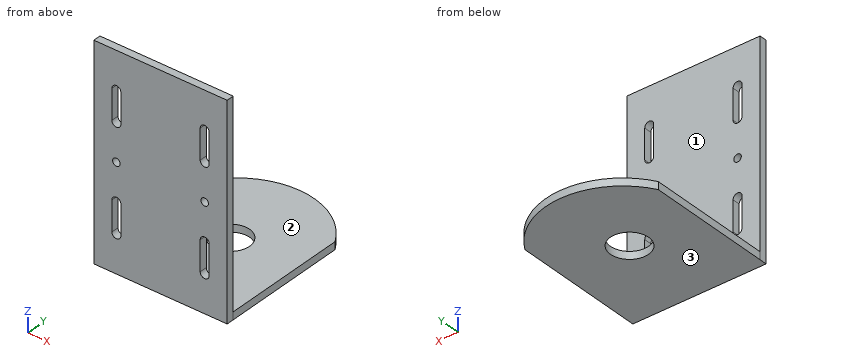
```python
from build123d import *

# Parameters (mm, degrees)
BOSS_EXTRUDE2_DEPTH = 10
BOSS_EXTRUDE3_DEPTH = 10
SKETCH2_R           = 25.4
CUT_EXTRUDE2_DEPTH  = 373.037550256
CUT_EXTRUDE5_DEPTH  = 10
SKETCH4_R           = 5
CUT_EXTRUDE6_DEPTH  = 366.966927049


with BuildPart() as part:
    # 3DSketch1 → Boss-Extrude2 (new body)
    with BuildSketch(Plane(origin=(88.9, 0, 0), x_dir=(-0.5368754921931593, 0, 0.8436614877321076), z_dir=(0, 1, 0))):
        Polygon((0, 0), (235.719019672, 150.003012519), (331.175482184, 0), (95.456462512, -150.003012519), align=None)
    extrude(amount=BOSS_EXTRUDE2_DEPTH)

    # Sketch1 → Boss-Extrude3 (add)
    with BuildSketch(Plane.XY):
        with BuildLine():
            Line((-88.9, 0), (88.9, 0))
            Line((88.9, 0), (88.9, 177.796999188))
            ThreePointArc((88.9, 177.796999188), (0, 229.007355341), (-88.9, 177.796999188))
            Line((-88.9, 177.796999188), (-88.9, 0))
        make_face()
    extrude(amount=BOSS_EXTRUDE3_DEPTH)

    # Sketch2 → Cut-Extrude2 (cut, through all)
    with BuildSketch(Plane(origin=(0, 0, 0), x_dir=(-1, 0, 0), z_dir=(0, 0, -1))):
        with Locations((0, 115.3)):
            Circle(SKETCH2_R)
    extrude(amount=-CUT_EXTRUDE2_DEPTH, mode=Mode.SUBTRACT)

    # Sketch3 → Cut-Extrude5 (cut)
    with BuildSketch(Plane(origin=(0, 10, 0), x_dir=(1, 0, 0), z_dir=(0, 1, 0))):
        with BuildLine():
            Line((-64.9, -90), (-64.9, -50))
            ThreePointArc((-64.9, -50), (-58.9, -44), (-52.9, -50))
            Line((-52.9, -50), (-52.9, -90))
            ThreePointArc((-52.9, -90), (-58.9, -96), (-64.9, -90))
        make_face()
        with BuildLine():
            Line((64.9, -90), (64.9, -50))
            ThreePointArc((64.9, -50), (58.9, -44), (52.9, -50))
            Line((52.9, -50), (52.9, -90))
            ThreePointArc((52.9, -90), (58.9, -96), (64.9, -90))
        make_face()
        with BuildLine():
            Line((64.9, -189.4), (64.9, -229.4))
            ThreePointArc((64.9, -229.4), (58.9, -235.4), (52.9, -229.4))
            Line((52.9, -229.4), (52.9, -189.4))
            ThreePointArc((52.9, -189.4), (58.9, -183.4), (64.9, -189.4))
        make_face()
        with BuildLine():
            Line((-64.9, -189.4), (-64.9, -229.4))
            ThreePointArc((-64.9, -229.4), (-58.9, -235.4), (-52.9, -229.4))
            Line((-52.9, -229.4), (-52.9, -189.4))
            ThreePointArc((-52.9, -189.4), (-58.9, -183.4), (-64.9, -189.4))
        make_face()
    extrude(amount=-CUT_EXTRUDE5_DEPTH, mode=Mode.SUBTRACT)

    # Sketch4 → Cut-Extrude6 (cut, through all)
    with BuildSketch(Plane(origin=(0, 10, 0), x_dir=(1, 0, 0), z_dir=(0, 1, 0))):
        with Locations(Location((-58.9, -139.7, 0), (0, 0, 270))):
            Circle(SKETCH4_R)
        with Locations(Location((58.9, -139.7, 0), (0, 0, 270))):
            Circle(SKETCH4_R)
    extrude(amount=-CUT_EXTRUDE6_DEPTH, mode=Mode.SUBTRACT)


solid = part.part
```
Part model, mm, in its own coordinate system. Face numbers are marked on the shaded views. Give positions to 0.01 mm unless a question says otherwise; leave off trailing zeros. Write each loop counter-clockwise with the first axis right and the second up, starting at its lowest first coordinate (ties: lowest second). Pieces come first, ordered by that corner, then holes. Notation, with made-up numbers: M -39.75,47 L -26.75,47 A28 ccw -26.75,65 Z; hole C -34,46.25 d1. An arc over 180 degrees is marked long. Use CSV: the item, a comma, the result in double quotes.
Item 1: Drill centre lines: probe 1 along X at (y, z) = (2.75, 139.7); probe 2 along Z at (x, y) = (-58, 8); probe 3 along Z at (x, y) = (-34.5, 146). Where is each one in solid material? Low to high.
Taken from the geometry:
probe 1,"x = -88.9 to -63.9, -53.9 to 53.9, 63.9 to 88.9"
probe 2,"z = 0 to 44.07, 95.93 to 134.78, 144.62 to 183.47, 235.33 to 279.4"
probe 3,"z = 0 to 10"
Item 2: Slice it at D-D on x = -58.9. Write the cut outline in (y, z), plus the area to 3 significant figures.
Taken from the geometry:
outline,"M 0,0 L 210.45,0 L 210.45,10 L 10,10 L 10,44 L 0,44 Z; M 0,96 L 10,96 L 10,134.7 L 0,134.7 Z; M 0,144.7 L 10,144.7 L 10,183.4 L 0,183.4 Z; M 0,235.4 L 10,235.4 L 10,279.4 L 0,279.4 Z"
area,"3,660 mm²"
Item 3: Slice it at B-B on x = 0. Write the cut outline in (y, z), plus the area to 3 significant figures.
Taken from the geometry:
outline,"M 0,0 L 89.9,0 L 89.9,10 L 10,10 L 10,279.4 L 0,279.4 Z; M 140.7,0 L 229.01,0 L 229.01,10 L 140.7,10 Z"
area,"4,480 mm²"
Item 4: Slice it at C-C on z = 139.7. Write the cut outline in (x, y), plus the area to 3 significant figures.
Taken from the geometry:
outline,"M -88.9,0 L -63.9,0 L -63.9,10 L -88.9,10 Z; M -53.9,0 L 53.9,0 L 53.9,10 L -53.9,10 Z; M 63.9,0 L 88.9,0 L 88.9,10 L 63.9,10 Z"
area,"1,580 mm²"
Item 5: Slice it at A-A on z = 70. Write the cut outline in (x, y), plus the area to 3 significant figures.
Taken from the geometry:
outline,"M -88.9,0 L -64.9,0 L -64.9,10 L -88.9,10 Z; M -52.9,0 L 52.9,0 L 52.9,10 L -52.9,10 Z; M 64.9,0 L 88.9,0 L 88.9,10 L 64.9,10 Z"
area,"1,540 mm²"
Item 6: Pin check, flat tips, straight feed: P1, Ø3, axis at x = 27.5, z = 99, coming from the +Y side; P2, Ø5, axis at x = 19, y = 90.5, coming from the +Z side; P3, Ø9, axis at x = -58.9, z = 139.7, coming from the +Y side. Stop position of each tip, or through.
Taken from the geometry:
P1,"stops at y = 10"
P2,"stops at z = 10"
P3,"passes through"
Item 7: Pull direction Z, two halves, no side cores. Call the marked faces 1, 2 and 3: +Z half, -Z half, draft (parallel to the pull), parting line (faces both ways), or undercut.
Taken from the geometry:
face 1,"draft"
face 2,"+Z half"
face 3,"-Z half"
